from build123d import *

# Parameters (mm, degrees)
F0_W     = 42
F0_H     = 42
F1_DEPTH = 400
F2_R     = 7.5
F3_DEPTH = 50
F4_W     = 42
F4_H     = 42
F5_DEPTH = 5
F6_R     = 2.5
F7_DEPTH = 50


with BuildPart() as f1:
    # F0 (on Top) → F1 (new body)
    with BuildSketch(Plane.XY):
        with BuildLine():
            Line((43.5, 46), (-1.5, 46))
            ThreePointArc((-1.5, 46), (-3.267767, 45.267767), (-4, 43.5))
            Line((-4, 43.5), (-4, -1.5))
            ThreePointArc((-4, -1.5), (-3.267767, -3.267767), (-1.5, -4))
            Line((-1.5, -4), (43.5, -4))
            ThreePointArc((43.5, -4), (45.267767, -3.267767), (46, -1.5))
            Line((46, -1.5), (46, 43.5))
            ThreePointArc((46, 43.5), (45.267767, 45.267767), (43.5, 46))
        make_face()
        with Locations((21, 21)):
            Rectangle(F0_W, F0_H, mode=Mode.SUBTRACT)
    extrude(amount=F1_DEPTH)

    # F2 (on face) → F3 (cut)
    with BuildSketch(Plane.XZ.offset(4)):
        with Locations((21, 380)):
            Circle(F2_R)
    extrude(amount=-F3_DEPTH, mode=Mode.SUBTRACT)

    # F4 (on face) → F5 (join)
    with BuildSketch(Plane.XY.offset(400)):
        with Locations((21, 21)):
            Rectangle(F4_W, F4_H)
    extrude(amount=-F5_DEPTH)

    # F6 (on face) → F7 (cut)
    with BuildSketch(Plane.XZ.offset(4)):
        with Locations((21, 324)):
            Circle(F6_R)
    extrude(amount=-F7_DEPTH, mode=Mode.SUBTRACT)


solid = f1.part
Check sheet for the modelled part. Datum: model origin and axes. Units: mm. A direction names the side the tool comes from. Give positions to 0.01 mm unless a question says otherwise; leave off trailing zeros. Write each loop counter-clockwise with the first axis right and the second up, starting at its lowest first coordinate (ties: lowest second). Pieces come first, ordered by that corner, then holes. Notation, with made-up numbers: (82, 50.5) -> (139, 50.5) arc R25 ccw to (139, 66.5) -> close; hole circle Ø2 at (19.5, 20). An arc over 180 degrees is marked (long way). One line per item, written item: value. Start each with the question number.
Item 1: Section check A-A on z = 380. Record the cut outline in (x, y), then the cut area to 3 significant figures.
Item 2: Draft check along X on faces 1 (the flat face through (21, 42, 195)), 2 (the cylindrical face through (19.37, -2.03, 372.68)), 3 (the flat face through (21, 44, 0)), 4 (the flat face through (-4, 21, 197)). Enter one of: +X half, -X half, draft (parallel to the pull), parting line (faces both ways), or undercut.
Item 3: Tool access check on faces 5 (the flat face through (42, 21, 195)), 6 (the flat face through (21, 21, 400)). Record the directions out of +Z, -Z, +X, -X, +Y, -Y that give a thin tool (end or side, any length) a straight path to the whole face; none if there is none.
Item 4: Section check D-D on z = 78.5. Record the cut outline in (x, y).
Item 5: Section check B-B on x = 35. Record the cut outline in (y, z), then the cut area to 3 significant figures.
Item 6: Material ranges on probe 1 along Y at (x, z) = (11, 263.5); probe 2 along Z at (x, y) = (21, 44.55), recorded low to high. Write a range as from..to.
Results list:
1. outline: (-4, -1.5) arc R2.5 ccw to (-1.5, -4) -> (13.5, -4) -> (13.5, 0) -> (0, 0) -> (0, 42) -> (13.5, 42) -> (13.5, 46) -> (-1.5, 46) arc R2.5 ccw to (-4, 43.5) -> close; (28.5, -4) -> (43.5, -4) arc R2.5 ccw to (46, -1.5) -> (46, 43.5) arc R2.5 ccw to (43.5, 46) -> (28.5, 46) -> (28.5, 42) -> (42, 42) -> (42, 0) -> (28.5, 0) -> close
1. area: 611 mm²
2. face 1: undercut
2. face 2: undercut
2. face 3: draft
2. face 4: -X half
3. face 5: -Z
3. face 6: +Z, +X, -X, +Y, -Y
4. outline: (-4, -1.5) arc R2.5 ccw to (-1.5, -4) -> (43.5, -4) arc R2.5 ccw to (46, -1.5) -> (46, 43.5) arc R2.5 ccw to (43.5, 46) -> (-1.5, 46) arc R2.5 ccw to (-4, 43.5) -> close; hole (0, 0) -> (42, 0) -> (42, 42) -> (0, 42) -> close
5. outline: (-4, 0) -> (0, 0) -> (0, 395) -> (42, 395) -> (42, 0) -> (46, 0) -> (46, 400) -> (-4, 400) -> close
5. area: 3,410 mm²
6. probe 1: -4..0, 42..46
6. probe 2: 0..321.5, 326.5..372.5, 387.5..400
